Could you check a few things on this model? Use its own coordinates, in mm. Face numbers are marked on the shaded views. Coordinates: 2 decimals unless noted, no trailing zeros. Loops run counter-clockwise (first coordinate to the right, second up) from the corner with the lowest first, then second, coordinate; pieces in that order, holes last. Notation, with made-up numbers: (-1, -2) -> (29, -2) arc R20 ccw to (29, 17) -> close; hole circle Ø2 at (42, 3.5). An arc over 180 degrees is marked (long way). One line per question, with ' | ' between items.
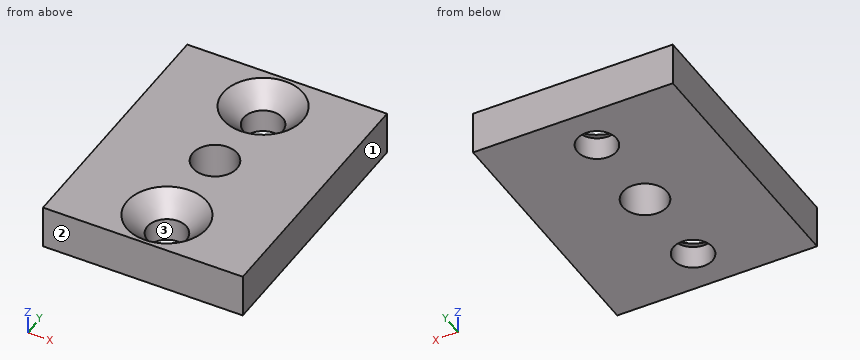
```python
from build123d import *

# Parameters (mm, degrees)
SKIZZE1_W                                            = 23
SKIZZE1_H                                            = 30
AUFSATZ_LINEAR_AUSTRAGEN1_DEPTH                      = 5
FORMSENKUNG_F_R_M4_SENKSCHRAUBE_MIT_INNE_D           = 4.5
FORMSENKUNG_F_R_M4_SENKSCHRAUBE_MIT_INNE_CSINK_D     = 9.18
FORMSENKUNG_F_R_M4_SENKSCHRAUBE_MIT_INNE_CSINK_ANGLE = 90
F_1_4_20_GEWINDEBOHRUNG1_D                           = 5.1054


with BuildPart() as part:
    # Skizze1 → Aufsatz-Linear austragen1 (new body)
    with BuildSketch(Plane.XY):
        with Locations((11.5, 15)):
            Rectangle(SKIZZE1_W, SKIZZE1_H)
    extrude(amount=AUFSATZ_LINEAR_AUSTRAGEN1_DEPTH)

    # Formsenkung für M4 Senkschraube mit Innensechskant1 (through all)
    with Locations(Plane.XY.offset(5)):
        with Locations((11.5, 25), (11.5, 5)):
            CounterSinkHole(FORMSENKUNG_F_R_M4_SENKSCHRAUBE_MIT_INNE_D / 2, FORMSENKUNG_F_R_M4_SENKSCHRAUBE_MIT_INNE_CSINK_D / 2, counter_sink_angle=FORMSENKUNG_F_R_M4_SENKSCHRAUBE_MIT_INNE_CSINK_ANGLE)

    # 1/4-20 Gewindebohrung1 (through all)
    with Locations(Plane.XY.offset(5)):
        with Locations((11.5, 15)):
            Hole(F_1_4_20_GEWINDEBOHRUNG1_D / 2)


solid = part.part
```
Q1. Imagine slicing it at C-C on z = 2.05. Write out the boundary of the cut face in (x, y).
Values follow:
outline: (0, 0) -> (23, 0) -> (23, 30) -> (0, 30) -> close; hole circle Ø5.11 at (11.5, 15); hole circle Ø4.5 at (11.5, 5); hole circle Ø4.5 at (11.5, 25)
Q2. Please list where these lines run through material, in increasing order: L1, parallel to Y at x = 11.5, z = 1.8; L2, parallel to X at y = 25, z = 0.9; L3, parallel to X at y = 22.5, z = 4.1. Write a range as [from, to].
Values follow:
L1: y = [0, 2.75], [7.25, 12.45], [17.55, 22.75], [27.25, 30] | L2: x = [0, 9.25], [13.75, 23] | L3: x = [0, 8.79], [14.21, 23]
Q3. Imagine slicing it at B-B on y = 25. Write out the boundary of the cut face in (x, z).
Values follow:
outline: (0, 0) -> (9.25, 0) -> (9.25, 2.66) -> (6.91, 5) -> (0, 5) -> close; (13.75, 0) -> (23, 0) -> (23, 5) -> (16.09, 5) -> (13.75, 2.66) -> close
Q4. We'd pull the mould along Y, two halves only. Please class the marked faces 1, 2 and 3: released by +Y, released by -Y, zero draft, split by the parting line, or undercut.
Values follow:
face 1: zero draft | face 2: released by -Y | face 3: undercut
Q5. Imagine slicing it at A-A on x = 11.5. Write out the boundary of the cut face in (y, z).
Values follow:
outline: (0, 0) -> (2.75, 0) -> (2.75, 2.66) -> (0.41, 5) -> (0, 5) -> close; (7.25, 0) -> (12.45, 0) -> (12.45, 5) -> (9.59, 5) -> (7.25, 2.66) -> close; (17.55, 0) -> (22.75, 0) -> (22.75, 2.66) -> (20.41, 5) -> (17.55, 5) -> close; (27.25, 0) -> (30, 0) -> (30, 5) -> (29.59, 5) -> (27.25, 2.66) -> close
Q6. Imagine slicing it at D-D on y = 15. Write out the boundary of the cut face in (x, z), plus the area to 3 significant figures.
Values follow:
outline: (0, 0) -> (8.95, 0) -> (8.95, 5) -> (0, 5) -> close; (14.05, 0) -> (23, 0) -> (23, 5) -> (14.05, 5) -> close | area: 89.5 mm2
Q7. For pin 1 (6 mm diameter, centred on x = 11.5, y = 5, fed in from +Z); pin 2 (7 mm diameter, centred on x = 11.5, y = 25, fed in from +Z), each with a flat end and sliding along its axis, tell me the tip position at first contact or that it passes through.
Values follow:
pin 1: stops at z = 3.41 | pin 2: stops at z = 3.91
